Input: part model. Units: mm. Frame: model coordinates. Face numbers are marked on the shaded views. A direction names the side the tool comes from. Round coordinates to 2 decimals unless told otherwise and drop trailing zeros. Loops run counter-clockwise (first coordinate to the right, second up) from the corner with the lowest first, then second, coordinate; pieces in that order, holes last. Notation, with made-up numbers: M 65.25,-18.5 L 124.25,-18.5 A24 ccw 124.25,16.5 Z; hole C 17.25,30.5 d8. An arc over 180 degrees is marked long. Return JSON: item names as keys, results as strings. Group by question number.
1) Section B-B (y = 34). Output: boundary loops of the cut face in (x, z).
2) Section C-C (x = 205). Output: boundary loops of the cut face in (y, z).
3) Section A-A (y = -14). Output: boundary loops of the cut face in (x, z).
4) Section D-D (z = -101). Output: boundary loops of the cut face in (x, y).
5) Access query for the marked faces 1 and 2. Directions: +Z, -Z, +X, -X, +Y, -Y. A direction counts if a zero-diameter tool reaches every point of the face in a straight line with its end or side. Return the directions, or none.
6) Contact query for flat-ended pins moving along their axis: P1, Ø6, axis at x = 196, z = -120.5, coming from the +Y side; P2, Ø18.5, axis at x = -108.82, y = 34, coming from the -Z side. Output: stop coordinate, or through.
7) Material intervals for line 1 (Z direction, x = 197.5, y = 57.5); line 2 (Y direction, x = 43, z = -49), sorted ascending. Write a range as from..to.
from build123d import *

# Parameters (mm, degrees)
SKETCH1_W           = 400
SKETCH1_H           = 108
BOSS_EXTRUDE1_DEPTH = 65
SKETCH3_W           = 400
SKETCH3_H           = 102
CUT_EXTRUDE1_DEPTH  = 158
SKETCH4_R           = 8
CUT_EXTRUDE2_DEPTH  = 158
SKETCH6_W           = 400
SKETCH6_H           = 3
BOSS_EXTRUDE3_DEPTH = 50
SKETCH7_W           = 400
SKETCH7_H           = 3
BOSS_EXTRUDE4_DEPTH = 102
SKETCH11_R          = 2.7
CUT_EXTRUDE4_DEPTH  = 75
SKETCH10_R          = 2.75
CUT_EXTRUDE3_DEPTH  = 75


with BuildPart() as part:
    # Sketch1 → Boss-Extrude1 (new body)
    with BuildSketch(Plane(origin=(0, 0, 0), x_dir=(1, 0, 0), z_dir=(0, 1, 0))):
        with Locations((66.180492252, 90.484958979)):
            Rectangle(SKETCH1_W, SKETCH1_H)
    extrude(amount=BOSS_EXTRUDE1_DEPTH)

    # Sketch3 → Cut-Extrude1 (cut)
    with BuildSketch(Plane.XZ):
        with Locations((66.180492252, -90.484958979)):
            Rectangle(SKETCH3_W, SKETCH3_H)
    extrude(amount=-CUT_EXTRUDE1_DEPTH, mode=Mode.SUBTRACT)


with BuildPart() as cut_extrude1_piece_1:
    # of the separate pieces the step leaves, piece 1, a body of its own (cut_extrude1_pieces)
    add(part.part.solids().sort_by_distance((-133.819507748, 0, -144.484958979))[0])


with BuildPart() as cut_extrude1_piece_2:
    # of the separate pieces the step leaves, piece 2, a body of its own (cut_extrude1_pieces)
    add(part.part.solids().sort_by_distance((-133.819507748, 0, -36.484958979))[0])


with BuildPart() as cut_extrude2_tool:
    # Sketch4 → Cut-Extrude2 (new body)
    with BuildSketch(Plane.XY.offset(-36.484958979)):
        with Locations((-108.819507748, 34)):
            Circle(SKETCH4_R)
        with Locations((241.180492252, 34)):
            Circle(SKETCH4_R)
    extrude(amount=-CUT_EXTRUDE2_DEPTH)


with BuildPart() as cut_extrude1_piece_1_1:
    add(cut_extrude1_piece_1.part)

    # Cut-Extrude2: cut by cut_extrude2_tool
    add(cut_extrude2_tool.part, mode=Mode.SUBTRACT)



with BuildPart() as cut_extrude1_piece_2_1:
    add(cut_extrude1_piece_2.part)

    # Cut-Extrude2: cut by cut_extrude2_tool
    add(cut_extrude2_tool.part, mode=Mode.SUBTRACT)


with BuildPart() as cut_extrude1_piece_1_2:
    add(cut_extrude1_piece_1_1.part)

    add(cut_extrude1_piece_2_1.part)  # Boss-Extrude3 merges Cut-Extrude1 piece 2
    # Sketch6 → Boss-Extrude3 (add)
    with BuildSketch(Plane.XZ):
        with Locations((66.180492252, -37.984958979)):
            Rectangle(SKETCH6_W, SKETCH6_H)
        with Locations((66.180492252, -142.984958979)):
            Rectangle(SKETCH6_W, SKETCH6_H)
    extrude(amount=BOSS_EXTRUDE3_DEPTH)

    # Sketch7 → Boss-Extrude4 (add)
    with BuildSketch(Plane(origin=(0, 0, -39.484958979), x_dir=(-1, 0, 0), z_dir=(0, 0, -1))):
        with Locations((-66.180492252, -48.5)):
            Rectangle(SKETCH7_W, SKETCH7_H)
    extrude(amount=BOSS_EXTRUDE4_DEPTH)

    # Sketch11 → Cut-Extrude4 (cut)
    with BuildSketch(Plane.XY.offset(-36.484958979)):
        with Locations((-33.819507748, -25.95)):
            Circle(SKETCH11_R)
    extrude(amount=-CUT_EXTRUDE4_DEPTH, mode=Mode.SUBTRACT)

    # Sketch10 → Cut-Extrude3 (cut)
    with BuildSketch(Plane(origin=(0, 0, -144.484958979), x_dir=(-1, 0, 0), z_dir=(0, 0, -1))):
        with Locations((-141.180492252, -28.85)):
            Circle(SKETCH10_R)
    extrude(amount=-CUT_EXTRUDE3_DEPTH, mode=Mode.SUBTRACT)


solid = cut_extrude1_piece_1_2.part
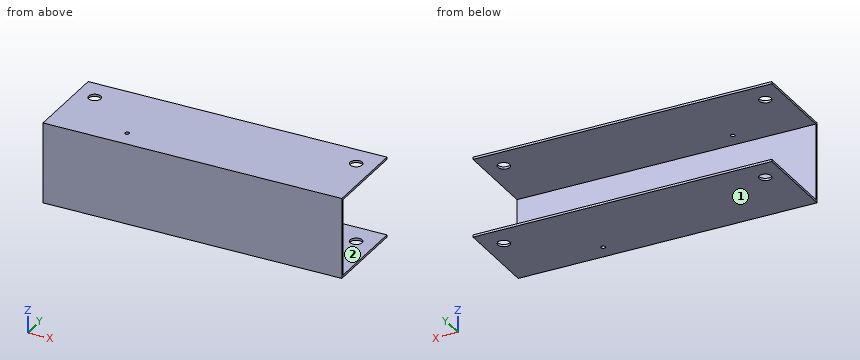
Returned:
{
 "1": {"outline": "M -133.82,-144.48 L -116.82,-144.48 L -116.82,-141.48 L -133.82,-141.48 Z; M -133.82,-39.48 L -116.82,-39.48 L -116.82,-36.48 L -133.82,-36.48 Z; M -100.82,-144.48 L 233.18,-144.48 L 233.18,-141.48 L -100.82,-141.48 Z; M -100.82,-39.48 L 233.18,-39.48 L 233.18,-36.48 L -100.82,-36.48 Z; M 249.18,-144.48 L 266.18,-144.48 L 266.18,-141.48 L 249.18,-141.48 Z; M 249.18,-39.48 L 266.18,-39.48 L 266.18,-36.48 L 249.18,-36.48 Z"},
 "2": {"outline": "M -50,-144.48 L 65,-144.48 L 65,-141.48 L -47,-141.48 L -47,-39.48 L 65,-39.48 L 65,-36.48 L -50,-36.48 Z"},
 "3": {"outline": "M -133.82,-144.48 L 266.18,-144.48 L 266.18,-141.48 L -133.82,-141.48 Z; M -133.82,-39.48 L 266.18,-39.48 L 266.18,-36.48 L -133.82,-36.48 Z"},
 "4": {"outline": "M -133.82,-50 L 266.18,-50 L 266.18,-47 L -133.82,-47 Z"},
 "5": {"face 1": "-Z, +X, -X, +Y, -Y", "face 2": "+X, -X, +Y"},
 "6": {"P1": "stops at y = -47", "P2": "stops at z = -144.48"},
 "7": {"line 1": "z = -144.48..-141.48, -39.48..-36.48", "line 2": "y = -50..-47"}
}
